Source: CAD feature listing. Evaluate the final solid. Frame: model axes, mm. Give positions to 0.01 mm unless a question says otherwise; leave off trailing zeros. Loops run counter-clockwise (first coordinate to the right, second up) from the corner with the lowest first, then second, coordinate; pieces in that order, holes last.
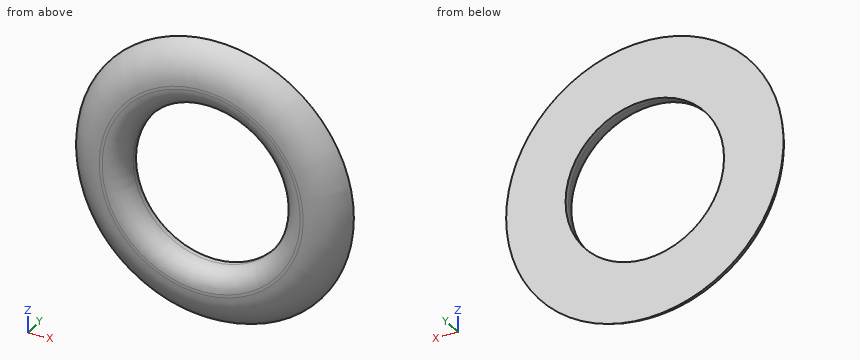
from build123d import *

# Parameters (mm, degrees)
F0_R     = 17.78
F0_R_2   = 10.16
F1_DEPTH = 3.175
F3_R     = 2.54


# Not quite as in the source:
# - a fillet or chamfer that OpenCascade refuses, or shapes differently, is made with other operations: its cross-section is extruded or revolved along the edge and cut away or added


with BuildPart() as f1:
    # F0 (on Front) → F1 (new body)
    with BuildSketch(Plane.XZ):
        Circle(F0_R)
        Circle(F0_R_2, mode=Mode.SUBTRACT)
    extrude(amount=F1_DEPTH)

    # F2: fillet of radius 5.08 on 1 edges, made by hand

    # F2_s1 → F2_t2 (revolve, cut)
    with BuildSketch(Plane.XY):
        with BuildLine():
            ThreePointArc((17.78, 0), (15.9105202921, -2.3071134838), (13.0707139607, -3.175))
            Line((13.0707139607, -3.175), (17.78, -3.175))
            Line((17.78, -3.175), (17.78, 0))
        make_face()
    revolve(axis=Axis((0, -3.175, 0), (0, -1, 0)), mode=Mode.SUBTRACT)

    # F3
    f3_edges = [f1.edges().sort_by_distance(p)[0] for p in [
        (-10.16, -3.175, 0),
    ]]
    fillet(f3_edges, radius=F3_R)


solid = f1.part
1) Contact query for flat-ended pins moving along their axis: P1, Ø10, axis at x = -2, z = -4, coming from the +Y side; P2, Ø8, axis at x = 4, z = 10.5, coming from the -Y side (3 decimals); P3, Ø1, axis at y = -1.5, z = 0, coming from the -X side. Output: stop coordinate, or through.
Checks:
P1: passes through
P2: stops at y = -3.175
P3: stops at x = -17.24
2) Ray query, probe 1 along Z at (x, y) = (0, -0.3); probe 2 along Z at (x, y) = (0, -1.15); probe 3 along X at (y, z) = (-2.65, -6.5). Return the intervals inside material, ascending.
Checks:
probe 1: z = -17.65 to -10.16, 10.16 to 17.65
probe 2: z = -17.13 to -10.21, 10.21 to 17.13
probe 3: x = -13.87 to -9.06, 9.06 to 13.87
3) Cut plane C-C (y = -1.45). Return loops of the section in (x, z), and give its area (3 significant figures).
Checks:
outline: circle Ø33.77 at (0, 0); hole circle Ø20.59 at (0, 0)
area: 563 mm2
4) Cut plane A-A (z = 0). Return loops of the section in (x, y) (3 decimals), and give its area (3 significant figures).
Checks:
outline: (-17.78, 0) arc R5.08 ccw to (-13.071, -3.175) - (-12.7, -3.175) arc R2.54 ccw to (-10.16, -0.635) - (-10.16, 0) - close; (10.16, -0.635) arc R2.54 ccw to (12.7, -3.175) - (13.071, -3.175) arc R5.08 ccw to (17.78, 0) - (10.16, 0) - close
area: 37.4 mm2
5) Cut plane B-B (x = 0). Return loops of the section in (y, z) (3 decimals), and give its area (3 significant figures).
Checks:
outline: (-3.175, -13.071) arc R5.08 ccw to (0, -17.78) - (0, -10.16) - (-0.635, -10.16) arc R2.54 ccw to (-3.175, -12.7) - close; (-3.175, 12.7) arc R2.54 ccw to (-0.635, 10.16) - (0, 10.16) - (0, 17.78) arc R5.08 ccw to (-3.175, 13.071) - close
area: 37.4 mm2
